from build123d import *

# Parameters (mm, degrees)
SKETCH1_W                 = 75
SKETCH1_H                 = 12.7
BOSS_EXTRUDE1_DEPTH       = 12.7
F_4_0MM_DOWEL_HOLE1_D     = 4
F_4_0MM_DOWEL_HOLE1_DEPTH = 117.6291
F_4_0MM_DOWEL_HOLE1_TIP   = 1.201721238
SKETCH4_W                 = 4
SKETCH4_H                 = 8
BOSS_EXTRUDE2_DEPTH       = 5
BOSS_EXTRUDE3_DEPTH       = 1


with BuildPart() as part:
    # Sketch1 → Boss-Extrude1 (new body)
    with BuildSketch(Plane(origin=(0, 0, 0), x_dir=(1, 0, 0), z_dir=(0, 1, 0))):
        with Locations((37.5, 6.35)):
            Rectangle(SKETCH1_W, SKETCH1_H)
    extrude(amount=BOSS_EXTRUDE1_DEPTH)

    # Ø4.0mm Dowel Hole1
    with Locations(Plane(origin=(0, 12.7, 0), x_dir=(1, 0, 0), z_dir=(0, 1, 0))):
        with Locations((69.5, 6.35), (59.5, 6.35), (5.5, 6.35), (15.5, 6.35)):
            Hole(F_4_0MM_DOWEL_HOLE1_D / 2, depth=F_4_0MM_DOWEL_HOLE1_DEPTH)
            with Locations((0, 0, -(F_4_0MM_DOWEL_HOLE1_DEPTH + F_4_0MM_DOWEL_HOLE1_TIP / 2))):  # 118° drill point
                Cone(0, F_4_0MM_DOWEL_HOLE1_D / 2, F_4_0MM_DOWEL_HOLE1_TIP, mode=Mode.SUBTRACT)

    # Sketch4 → Boss-Extrude2 (add)
    with BuildSketch(Plane.XY):
        with Locations((18, 6.35)):
            Rectangle(SKETCH4_W, SKETCH4_H)
    extrude(amount=BOSS_EXTRUDE2_DEPTH)

    # Sketch6 → Boss-Extrude3 (add)
    with BuildSketch(Plane(origin=(75, 0, 0), x_dir=(0, 0, -1), z_dir=(1, 0, 0))):
        Polygon((6.35, 0), (12.7, 12.7), (6.35, 6.35), (0, 12.7), align=None)
    extrude(amount=BOSS_EXTRUDE3_DEPTH)


solid = part.part
The model under review builds one solid part; all positions refer to its coordinate system, in mm. A direction names the side the tool comes from. Coordinates: 2 decimals unless noted, no trailing zeros. Write each loop counter-clockwise with the first axis right and the second up, starting at its lowest first coordinate (ties: lowest second). Pieces come first, ordered by that corner, then holes. Notation, with made-up numbers: M 71,1.5 L 94,1.5 A32 ccw 94,33.5 Z; hole C 21,67 d2. An arc over 180 degrees is marked long. Put each result on its own line as item: value.
1) Clearance check with flat-ended pins moving along their axes: pin 1 Ø3 at (y, z) = (9.5, -6.5) entering from +X; pin 2 Ø1.5 at (y, z) = (8.5, 1.5) entering from -X; pin 3 Ø2.5 at (y, z) = (7.5, 2) entering from +X. State where each tip first meets the part, or that it passes through.
Computed:
pin 1: stops at x = 75
pin 2: stops at x = 16
pin 3: stops at x = 20
2) Wall thickness on probe 1 along Z at (x, y) = (15.5, 9.75); probe 2 along X at (y, z) = (12.25, -6.75); probe 3 along X at (y, z) = (4.25, -5.75): over which ranges is each line inside the solid? List them lowest first. Write a range as [from, to].
Computed:
probe 1: z = [-12.7, -8.35], [-4.35, 0]
probe 2: x = [0, 3.54], [7.46, 13.54], [17.46, 57.54], [61.46, 67.54], [71.46, 75]
probe 3: x = [0, 3.59], [7.41, 13.59], [17.41, 57.59], [61.41, 67.59], [71.41, 76]
3) For faces 5 (the flat face through (20, 6, 2)), 6 (the flat face through (75, 5, -2)), 7 (the flat face through (75.5, 9.6, -9.6)), 8 (the flat face through (18, 2.35, 2)), list the 3-axis set-ups (+Z, -Z, +X, -X, +Y, -Y) from which the entire face can be reached by the end or side of a thin tool; tool diameter is ignored.
Computed:
face 5: +Z, +X, +Y, -Y
face 6: +Z, +X, -Y
face 7: +X, +Y
face 8: +Z, +X, -X, -Y
4) Add section D-D on y = 11.5. Give the boundary of the cut face in (x, z).
Computed:
outline: M 0,-12.7 L 75,-12.7 L 75,-12.1 L 76,-12.1 L 76,-11.5 L 75,-11.5 L 75,-1.2 L 76,-1.2 L 76,-0.6 L 75,-0.6 L 75,0 L 0,0 Z; hole C 5.5,-6.35 d4; hole C 15.5,-6.35 d4; hole C 59.5,-6.35 d4; hole C 69.5,-6.35 d4
5) Add section B-B on y = 5. Give the boundary of the cut face in (x, z), then the cut area to 3 significant figures.
Computed:
outline: M 0,-12.7 L 75,-12.7 L 75,-8.85 L 76,-8.85 L 76,-3.85 L 75,-3.85 L 75,0 L 20,0 L 20,5 L 16,5 L 16,0 L 0,0 Z; hole C 5.5,-6.35 d4; hole C 15.5,-6.35 d4; hole C 59.5,-6.35 d4; hole C 69.5,-6.35 d4
area: 927 mm2
6) Add section A-A on x = 69.5. Give the boundary of the cut face in (y, z), then the cut area to 3 significant figures.
Computed:
outline: M 0,-12.7 L 12.7,-12.7 L 12.7,-8.35 L 0,-8.35 Z; M 0,-4.35 L 12.7,-4.35 L 12.7,0 L 0,0 Z
area: 110 mm2
7) Add section C-C on x = 54.5. Give the boundary of the cut face in (y, z), then the cut area to 3 significant figures.
Computed:
outline: M 0,-12.7 L 12.7,-12.7 L 12.7,0 L 0,0 Z
area: 161 mm2
8) Draft analysis for pull direction X (two halves, no side actions). For faces 1 (the cylindrical face through (15.934, 6.261, -4.398)), 2 (the flat face through (16, 6, 2)), 3 (the cylindrical face through (67.592, 6.261, -6.951)), 4 (the flat face through (75.49, 6.44, -3.13)), state which applies: released by +X, released by -X, zero draft, split by the parting line, or undercut.
Computed:
face 1: undercut
face 2: released by -X
face 3: undercut
face 4: zero draft
